```python
from build123d import *

# Parameters (mm, degrees)
SKETCH2_R                = 25
BOSS_EXTRUDE1_DEPTH      = 45
BOSS_EXTRUDE2_DEPTH      = 45
BOSS_EXTRUDE2_DEPTH_BACK = 445
SKETCH2_3_R              = 25
CHAMFER1_SIZE            = 4


with BuildPart() as part:
    # Sketch2 → Boss-Extrude1 (new body)
    with BuildSketch(Plane(origin=(0, 0, 0), x_dir=(1, 0, 0), z_dir=(0, 1, 0))):
        Polygon((60.044427996, 0), (30.022213998, 52), (-30.022213998, 52), (-60.044427996, 0), (-30.022213998, -52), (30.022213998, -52), align=None)
        with Locations(Location((0, 0, 0), (0, 0, 90))):
            Circle(SKETCH2_R, mode=Mode.SUBTRACT)
    extrude(amount=BOSS_EXTRUDE1_DEPTH)

    # Sketch2_3 → Boss-Extrude2 (add, two sides: drawn at the far end of the back side and taken through both)
    with BuildSketch(Plane(origin=(0, 0, 0), x_dir=(1, 0, 0), z_dir=(0, 1, 0)).offset(-BOSS_EXTRUDE2_DEPTH_BACK)):
        with Locations(Location((0, 0, 0), (0, 0, 270))):
            Circle(SKETCH2_3_R)
    extrude(amount=BOSS_EXTRUDE2_DEPTH + BOSS_EXTRUDE2_DEPTH_BACK)

    # Chamfer1
    chamfer1_edges = [part.edges().sort_by_distance(p)[0] for p in [
        (0, -445, -25),
    ]]
    chamfer(chamfer1_edges, length=CHAMFER1_SIZE)


solid = part.part
```
Here's how the part is built. I have some questions about the finished solid (model axes, mm). A direction names the side the tool comes from. Round coordinates to 2 decimals unless told otherwise and drop trailing zeros. Order: outer loops, then holes, each group sorted by start corner. A loop starts at its lowest first (then second) coordinate and runs counter-clockwise, first axis right, second up. Notation, with made-up numbers: M 50,6.25 L 73,6.25 A24 cw 73,25.25 Z; hole C 62,35 d3. An arc over 180 degrees is marked long. Answer in a Markdown table with one row per item.
Item 1: For faces 4 (the face through (7.509, -223.587, 23.846)), 5 (the face through (45.24, 22.18, -25.64)), which set-ups out of +Z, -Z, +X, -X, +Y, -Y let a thin tool reach every point of the face, with its end or its side?
A:
| item | result |
|---|---|
| face 4 | -Y |
| face 5 | -Z, +X, +Y, -Y |
Item 2: If I drill on L1, parallel to Y at x = -21.5, z = 46; L2, parallel to Z at x = -7, y = -40; L3, parallel to X at y = 4, z = 10.5, over which ranges is the centre line in solid material (lowest first)? Write a range as from..to.
A:
| item | result |
|---|---|
| L1 | y = 0..45 |
| L2 | z = -24..24 |
| L3 | x = -53.98..53.98 |
Item 3: I'm going to push flat-ended pins straight in: pin 1 (4 mm diameter, centred on y = -75, z = -12, fed in from +X); pin 2 (4 mm diameter, centred on x = -3.5, z = 37, fed in from -Y); pin 3 (12 mm diameter, centred on y = -304, z = 3, fed in from -X). Where does each tip first touch, or does it pass through?
A:
| item | result |
|---|---|
| pin 1 | stops at x = 22.91 |
| pin 2 | stops at y = 0 |
| pin 3 | stops at x = -25 |
Item 4: Imagine slicing it at A-A, the plane x = 0. Write out the boundary of the cut face in (y, z), and give its area (3 significant figures).
A:
| item | result |
|---|---|
| outline | M -445,-21 L -441,-25 L 0,-25 L 0,-52 L 45,-52 L 45,52 L 0,52 L 0,25 L -441,25 L -445,21 Z |
| area | 26,900 mm2 |
Item 5: Imagine slicing it at B-B, the plane y = -338. Write out the boundary of the cut face in (x, z), and give its area (3 significant figures).
A:
| item | result |
|---|---|
| outline | C 0,0 d50 |
| area | 1,960 mm2 |
Item 6: Imagine slicing it at D-D, the plane x = -47. Write out the boundary of the cut face in (y, z).
A:
| item | result |
|---|---|
| outline | M 0,-22.59 L 45,-22.59 L 45,22.59 L 0,22.59 Z |
Item 7: Thinking about a two-plate mould opening in X: for faces 1 (the face through (44.823, 22.185, 26.364)), 2 (the face through (-44.823, 22.185, -26.364)), 3 (the face through (0, -445, 0)), which applies, +X half, -X half, draft (parallel to the pull), parting line (faces both ways), or undercut?
A:
| item | result |
|---|---|
| face 1 | +X half |
| face 2 | -X half |
| face 3 | draft |
Item 8: Imagine slicing it at C-C, the plane z = -39. Write out the boundary of the cut face in (x, y).
A:
| item | result |
|---|---|
| outline | M -37.53,0 L 37.53,0 L 37.53,45 L -37.53,45 Z |
